Check sheet for the drawn part. Datum: minimum x, y, z corner. Units: mm. Give positions to 0.01 mm unless a question says otherwise; leave off trailing zeros. Order: outer loops, then holes, each group sorted by start corner. A loop starts at its lowest first (then second) coordinate and runs counter-clockwise, first axis right, second up. Notation, with made-up numbers: (-38, 41.25) -> (-5, 41.25) arc R31 ccw to (-5, 67.25) -> close; hole circle Ø7 at (25, 62.5). An arc over 180 degrees is marked (long way). Answer in a Markdown table with one row per item. Add a question column.
(1) Go/stop test with flat-tipped pins: pin 1 (1.5 mm diameter, centred on x = 0.5, z = 22, fed in from -Y); pin 2 (1.5 mm diameter, centred on y = 5.5, z = 14, fed in from -X); pin 3 (0.5 mm diameter, centred on x = 2, y = 2, fed in from -Z). Record where each tip stops, or that it passes through.
(2) Cross-section at D-D (z = 11). Record the cut outline in (x, y).
(3) Cross-section at B-B (z = 4). Record the cut outline in (x, y).
(4) Thickness scan on L1, parallel to Y at x = 2.2, z = 2.5; L2, parallel to Y at x = 2, z = 3.8; L3, parallel to X at y = 7, z = 12. Record the ranges inside material, lowest first. Write a range as [from, to].
(5) Cross-section at C-C (y = 2). Record the cut outline in (x, z).
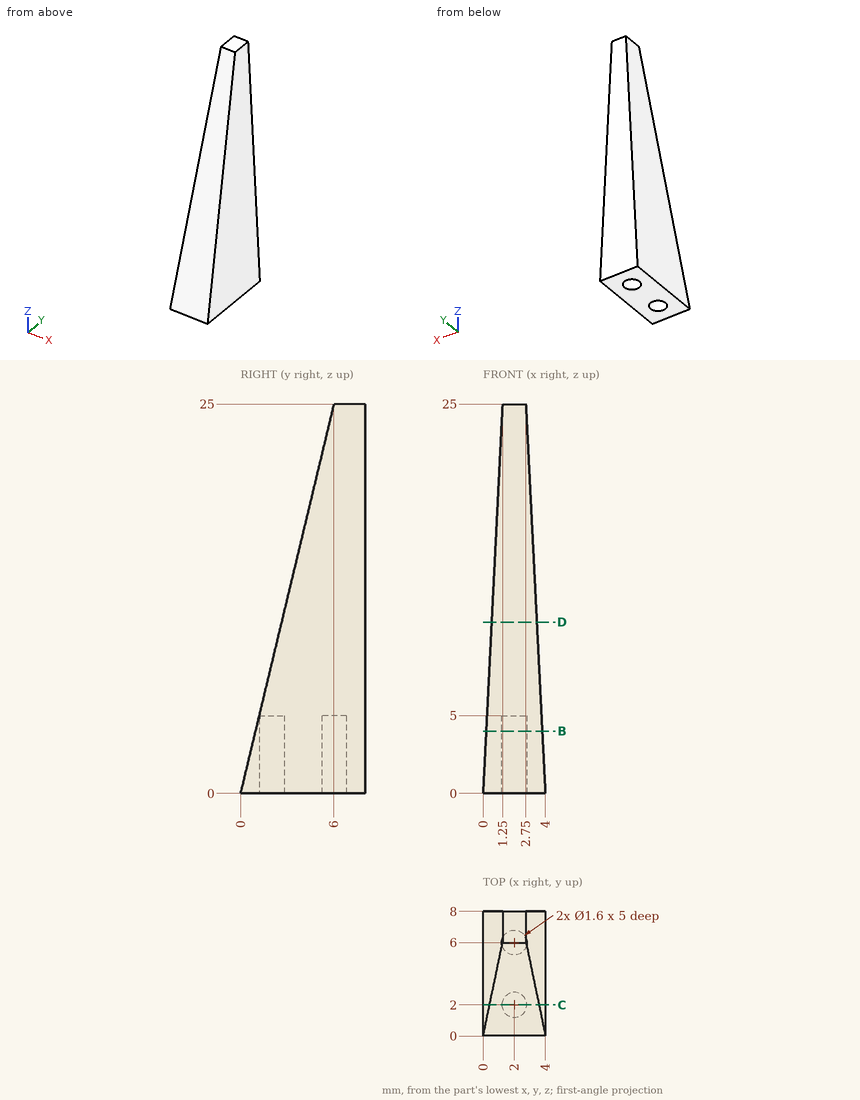
Answer below:
| question | item | result |
|---|---|---|
| 1 | pin 1 | stops at y = 5.16 |
| 1 | pin 2 | stops at x = 0.66 |
| 1 | pin 3 | stops at z = 5 |
| 2 | outline | (0.55, 2.64) -> (3.45, 2.64) -> (3.45, 8) -> (0.55, 8) -> close |
| 3 | outline | (0.2, 0.96) -> (3.8, 0.96) -> (3.8, 8) -> (0.2, 8) -> close; hole circle Ø1.6 at (2, 2); hole circle Ø1.6 at (2, 6) |
| 4 | L1 | y = [0.6, 1.23], [2.77, 5.23], [6.77, 8] |
| 4 | L2 | y = [0.91, 1.2], [2.8, 5.2], [6.8, 8] |
| 4 | L3 | x = [0.6, 3.4] |
| 5 | outline | (0, 0) -> (1.2, 0) -> (1.2, 5) -> (2.8, 5) -> (2.8, 0) -> (4, 0) -> (3.58, 8.33) -> (0.42, 8.33) -> close |
